```python
from build123d import *

# Parameters (mm, degrees)
SKETCH1_W           = 220
SKETCH1_H           = 230
BOSS_EXTRUDE1_DEPTH = 20
FILLET1_R           = 30
BOSS_EXTRUDE4_DEPTH = 10
CUT_EXTRUDE10_DEPTH = 20
SKETCH6_R           = 5.025
CUT_EXTRUDE3_DEPTH  = 31
SKETCH8_R           = 5
CUT_EXTRUDE4_DEPTH  = 30
SKETCH7_R           = 5
CUT_EXTRUDE5_DEPTH  = 30
CUT_EXTRUDE6_DEPTH  = 8.5
CUT_EXTRUDE7_DEPTH  = 8.5
CUT_EXTRUDE8_DEPTH  = 26.5
CUT_EXTRUDE9_DEPTH  = 31


with BuildPart() as part:
    # Sketch1 → Boss-Extrude1 (new body)
    with BuildSketch(Plane(origin=(0, 0, 0), x_dir=(1, 0, 0), z_dir=(0, 1, 0))):
        with Locations((110, 115)):
            Rectangle(SKETCH1_W, SKETCH1_H)
    extrude(amount=BOSS_EXTRUDE1_DEPTH)

    # Fillet1
    fillet1_edges = [part.edges().sort_by_distance(p)[0] for p in [
        (0, 10, -230),
        (220, 10, -230),
        (220, 10, 0),
        (0, 10, 0),
    ]]
    fillet(fillet1_edges, radius=FILLET1_R)

    # Sketch4 → Boss-Extrude4 (add)
    with BuildSketch(Plane(origin=(0, 0, 0), x_dir=(-1, 0, 0), z_dir=(0, -1, 0))):
        with BuildLine():
            Line((-225, 200), (-225, 30))
            ThreePointArc((-225, 30), (-214.748737342, 5.251262658), (-190, -5))
            Line((-190, -5), (-30, -5))
            ThreePointArc((-30, -5), (-5.251262658, 5.251262658), (5, 30))
            Line((5, 30), (5, 200))
            ThreePointArc((5, 200), (-5.251262658, 224.748737342), (-30, 235))
            Line((-30, 235), (-190, 235))
            ThreePointArc((-190, 235), (-214.748737342, 224.748737342), (-225, 200))
        make_face()
    extrude(amount=BOSS_EXTRUDE4_DEPTH)

    # Sketch15 → Cut-Extrude10 (cut)
    with BuildSketch(Plane(origin=(0, 20, 0), x_dir=(1, 0, 0), z_dir=(0, 1, 0))):
        with BuildLine():
            Line((215, 30), (215, 200))
            ThreePointArc((215, 200), (207.67766953, 217.67766953), (190, 225))
            Line((190, 225), (30, 225))
            ThreePointArc((30, 225), (12.32233047, 217.67766953), (5, 200))
            Line((5, 200), (5, 30))
            ThreePointArc((5, 30), (12.32233047, 12.32233047), (30, 5))
            Line((30, 5), (190, 5))
            ThreePointArc((190, 5), (207.67766953, 12.32233047), (215, 30))
        make_face()
    extrude(amount=-CUT_EXTRUDE10_DEPTH, mode=Mode.SUBTRACT)

    # Sketch6 → Cut-Extrude3 (cut, through all)
    with BuildSketch(Plane(origin=(0, -10, 0), x_dir=(-1, 0, 0), z_dir=(0, -1, 0))):
        with Locations((-200, 205)):
            Circle(SKETCH6_R)
        with Locations((-20, 205)):
            Circle(SKETCH6_R)
        with Locations((-20, 25)):
            Circle(SKETCH6_R)
        with Locations((-200, 25)):
            Circle(SKETCH6_R)
    extrude(amount=-CUT_EXTRUDE3_DEPTH, mode=Mode.SUBTRACT)

    # Sketch8 → Cut-Extrude4 (cut)
    with BuildSketch(Plane(origin=(0, 0, -230), x_dir=(-1, 0, 0), z_dir=(0, 0, -1))):
        with Locations((-150, 10)):
            Circle(SKETCH8_R)
        with Locations((-70, 10)):
            Circle(SKETCH8_R)
    extrude(amount=-CUT_EXTRUDE4_DEPTH, mode=Mode.SUBTRACT)

    # Sketch7 → Cut-Extrude5 (cut)
    with BuildSketch(Plane.XY):
        with Locations((70, 10)):
            Circle(SKETCH7_R)
        with Locations((150, 10)):
            Circle(SKETCH7_R)
    extrude(amount=-CUT_EXTRUDE5_DEPTH, mode=Mode.SUBTRACT)

    # Sketch10 → Cut-Extrude6 (cut)
    with BuildSketch(Plane(origin=(0, 0, -230), x_dir=(-1, 0, 0), z_dir=(0, 0, -1))):
        Polygon((-159.237604307, 10), (-154.618802154, 2), (-145.381197846, 2), (-140.762395693, 10), (-145.381197846, 18), (-154.618802154, 18), align=None)
        Polygon((-79.237604307, 10), (-74.618802154, 2), (-65.381197846, 2), (-60.762395693, 10), (-65.381197846, 18), (-74.618802154, 18), align=None)
    extrude(amount=-CUT_EXTRUDE6_DEPTH, mode=Mode.SUBTRACT)

    # Sketch9 → Cut-Extrude7 (cut)
    with BuildSketch(Plane.XY):
        Polygon((60.762395693, 10), (65.381197846, 2), (74.618802154, 2), (79.237604307, 10), (74.618802154, 18), (65.381197846, 18), align=None)
        Polygon((154.618802154, 2), (145.381197846, 2), (140.762395693, 10), (145.381197846, 18), (154.618802154, 18), (159.237604307, 10), align=None)
    extrude(amount=-CUT_EXTRUDE7_DEPTH, mode=Mode.SUBTRACT)

    # Sketch11 → Cut-Extrude8 (cut)
    with BuildSketch(Plane(origin=(0, 20, 0), x_dir=(1, 0, 0), z_dir=(0, 1, 0))):
        Polygon((20, 214.237604307), (12, 209.618802154), (12, 200.381197846), (20, 195.762395693), (28, 200.381197846), (28, 209.618802154), align=None)
        Polygon((192, 209.618802154), (200, 214.237604307), (208, 209.618802154), (208, 200.381197846), (200, 195.762395693), (192, 200.381197846), align=None)
        Polygon((192, 29.618802154), (192, 20.381197846), (200, 15.762395693), (208, 20.381197846), (208, 29.618802154), (200, 34.237604307), align=None)
        Polygon((28, 20.381197846), (20, 15.762395693), (12, 20.381197846), (12, 29.618802154), (20, 34.237604307), (28, 29.618802154), align=None)
    extrude(amount=-CUT_EXTRUDE8_DEPTH, mode=Mode.SUBTRACT)

    # Sketch13 → Cut-Extrude9 (cut, through all)
    with BuildSketch(Plane.XZ.offset(10)):
        with BuildLine():
            Line((135, -65), (85, -65))
            ThreePointArc((85, -65), (75, -55), (85, -45))
            Line((85, -45), (135, -45))
            ThreePointArc((135, -45), (145, -55), (135, -65))
        make_face()
    extrude(amount=-CUT_EXTRUDE9_DEPTH, mode=Mode.SUBTRACT)


solid = part.part
```
Design review of the part built by this model. Coordinates are the model's own, in mm. A direction names the side the tool comes from. Coordinates: 2 decimals unless noted, no trailing zeros. Order: outer loops, then holes, each group sorted by start corner. A loop starts at its lowest first (then second) coordinate and runs counter-clockwise, first axis right, second up. Notation, with made-up numbers: (-5, 68.25) -> (44, 68.25) arc R20 cw to (44, 95.25) -> close; hole circle Ø10 at (88.5, -16.75). An arc over 180 degrees is marked (long way). One line per item, written item: value. Start each with the question number.
Q1. Take a section at A-A, the plane z = -55. State the section outline as (x, y) points.
Q2. Take a section at D-D, the plane y = 15.25. Give the number of separate pieces and of enclosed holes in the cut face, then the cut area to 3 significant figures.
Q3. Take a section at C-C, the plane z = -171.5. State the section outline as (x, y) points, then the cut area to 3 significant figures.
Q4. Insertion check: pin 1 Ø5 at (y, z) = (-3.5, -206.5) entering from +X; pin 2 Ø6 at (y, z) = (7, -125.5) entering from +X; pin 3 Ø2 at (y, z) = (-3.5, -23.5) entering from +X. Each pin has a flat end and moves straight along its axis. Give the tip position at first contact, or say it passes through.
Q5. For probe 1 along Z at (x, y) = (127, -5.25); probe 2 along Z at (x, y) = (200, -8.5) (3 decimals); probe 3 along Z at (x, y) = (36.5, 5.25), list the stretches that pass through material, from the lowest coordinate up.
Q6. Tool access review of faces 5 (the flat face through (215, 10, -114)), 6 (the flat face through (109, 10, -230)): name each direction out of +Z, -Z, +X, -X, +Y, -Y from which nothing blocks a thin tool from reaching the whole face with its end or side.
Q7. Mouldability with a two-part tool opening along X and no side actions: class faces 1 (the flat face through (111, 0, -231)), 2 (the flat face through (225, -5, -116)), 3 (the flat face through (196.056, -3.204, -198.039)), 4 (the cylindrical face through (195.358, -8.274, -203.075)) as pulls with the +X half, pulls with the -X half, needs draft (parallel to the pull), parting line crosses it, or undercut.
Q8. Take a section at B-B, the plane x = 110. State the section outline as (y, z) points, then the cut area to 3 significant figures.
Values follow:
1. outline: (-5, -10) -> (75, -10) -> (75, 0) -> (5, 0) -> (5, 20) -> (0, 20) -> (0, 0) -> (-5, 0) -> close; (145, -10) -> (225, -10) -> (225, 0) -> (220, 0) -> (220, 20) -> (215, 20) -> (215, 0) -> (145, 0) -> close
2. separate pieces: 4
2. enclosed holes: 0
2. area: 3,920 mm2
3. outline: (-5, -10) -> (225, -10) -> (225, 0) -> (220, 0) -> (220, 20) -> (215, 20) -> (215, 0) -> (5, 0) -> (5, 20) -> (0, 20) -> (0, 0) -> (-5, 0) -> close
3. area: 2,500 mm2
4. pin 1: stops at x = 224.77
4. pin 2: stops at x = 220
4. pin 3: stops at x = 224.57
5. probe 1: z = -235 to -65, -45 to 5
5. probe 2: z = -233.541 to -210.025, -199.975 to -30.025, -19.975 to 3.541
5. probe 3: z = -230 to -225, -5 to 0
6. face 5: +Y
6. face 6: -Z, +X, -X, +Y
7. face 1: needs draft
7. face 2: pulls with the +X half
7. face 3: undercut
7. face 4: undercut
8. outline: (-10, -235) -> (0, -235) -> (0, -230) -> (20, -230) -> (20, -225) -> (0, -225) -> (0, -65) -> (-10, -65) -> close; (-10, -45) -> (0, -45) -> (0, -5) -> (20, -5) -> (20, 0) -> (0, 0) -> (0, 5) -> (-10, 5) -> close
8. area: 2,400 mm2
